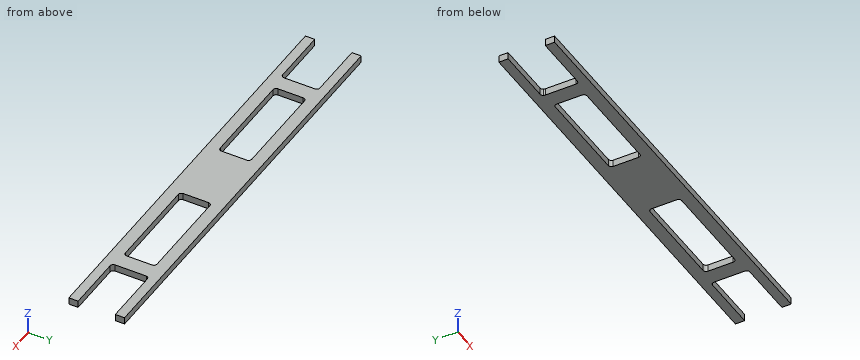
Autodesk Inventor part; units mm, degrees
ref_plane "YZ Plane" through (0, 0, 0) normal (1, 0, 0) x (0, 1, 0)
ref_plane "XZ Plane" through (0, 0, 0) normal (0, 1, 0) x (-1, 0, 0)
ref_plane "XY Plane" through (0, 0, 0) normal (0, 0, 1) x (1, 0, 0)
sketch "Sketch1" plane through (0, 0, 0) normal (0, 0, 1) x (1, 0, 0)
  line L0 (282.4312, 43.9885) -> (-286.5277, 43.9885)
  line L1 (-286.5288, -32.1915) -> (282.4312, -32.1915)
  line L2 (-286.5277, 43.9885) -> (-286.5277, 31.2885)
  line L3 (-286.5288, -19.4915) -> (-286.5288, -32.1915)
  line L4 (282.4312, 31.3086) -> (282.4312, 43.9885)
  line L5 (282.4312, -19.4915) -> (282.4312, -32.1915)
  arc A0 (-205.7269, 29.0424) -> (-209.4741, 31.2885) centre (-209.4741, 27.0395) ccw
  arc A1 (-205.2441, 26.6389) -> (-205.7269, 29.0424) centre (-209.4741, 27.0395) ccw
  arc A2 (-209.4751, -19.4915) -> (-205.2441, -15.2625) centre (-209.4741, -15.2615) ccw
  arc A3 (-179.9924, 27.4418) -> (-183.6588, 23.2495) centre (-179.4288, 23.2495) ccw
  arc A4 (-183.6588, -11.4325) -> (-179.4288, -15.6625) centre (-179.4288, -11.4325) ccw
  arc A5 (-48.2006, 23.2495) -> (-52.4306, 27.4418) centre (-52.4304, 23.2118) ccw
  arc A6 (-52.9924, -15.6625) -> (-48.2006, -11.4325) centre (-52.4304, -11.47) ccw
  line L6 (-52.4306, 27.4418) -> (-179.9924, 27.4418)
  line L7 (-52.9924, -15.6625) -> (-179.4288, -15.6625)
  line L8 (-48.2006, -11.4325) -> (-48.2006, 23.2495)
  line L9 (-183.6588, -11.4325) -> (-183.6588, 23.2495)
  arc A7 (205.3642, 31.3086) -> (201.1322, 27.4399) centre (205.3642, 27.0596) ccw
  arc A8 (201.1322, -15.2425) -> (205.3812, -19.4915) centre (205.3812, -15.2425) ccw
  line L10 (201.1322, -15.2425) -> (201.1322, 23.2474)
  line L11 (201.1322, 23.2474) -> (201.1322, 27.4399)
  line L12 (282.4312, 31.3086) -> (205.3642, 31.3086)
  line L13 (282.4312, -19.4915) -> (205.3812, -19.4915)
  line L14 (-286.5288, -19.4915) -> (-209.4751, -19.4915)
  line L15 (-286.5277, 31.2885) -> (-209.4741, 31.2885)
  line L16 (-205.2441, 26.6389) -> (-205.2441, -15.2625)
  arc A9 (48.2152, 27.4415) -> (43.9852, 23.2115) centre (48.2152, 23.2115) ccw
  arc A10 (43.9852, -11.4145) -> (48.2152, -15.6445) centre (48.2152, -11.4145) ccw
  arc A11 (179.5472, 23.2115) -> (175.3172, 27.4415) centre (175.3172, 23.2115) ccw
  arc A12 (175.3172, -15.6445) -> (179.5472, -11.4145) centre (175.3172, -11.4145) ccw
  line L17 (48.2152, 27.4415) -> (175.3172, 27.4415)
  line L18 (48.2152, -15.6445) -> (175.3172, -15.6445)
  line L19 (43.9852, 23.2115) -> (43.9852, -11.4145)
  line L20 (179.5472, 23.2115) -> (179.5472, -11.4145)
  point P0 (0, 0)
  point P1 (0, 0)
  dimension "d0" = 135.4582
  dimension "d1" = 43.1043
  dimension "d2" = 16.5467
  dimension "d3" = 16.529
  dimension "d4" = 21.5853
  dimension "d5" = 92.1858
extrude "Extrusion1" add sketch "Sketch1" along normal blind 9.525
properties part number "top"
Design review of the part built by this model. Coordinates are the model's own, in mm. Coordinates: 2 decimals unless noted, no trailing zeros. Loops run counter-clockwise (first coordinate to the right, second up) from the corner with the lowest first, then second, coordinate; pieces in that order, holes last. Notation, with made-up numbers: M 74.25,36.25 L 83.25,36.25 A30 cw 83.25,67.25 Z; hole C 51.25,42.5 d11. An arc over 180 degrees is marked long. Answer as CSV lines item,"result".
Item 1: For P1, Ø3, axis at y = 1, z = 3.5, coming from the -X side; P2, Ø5, axis at y = 13.5, z = 7.5, coming from the +X side, all flat-tipped, find the tip position at first contact; note any pin that passes through.
Answer list:
P1,"x = -205.24"
P2,"x = 201.13"
Item 2: Add section A-A on y = 8. State the section outline as (x, z) points (3 decimals), plus the area to 3 significant figures.
Answer list:
outline,"M -205.244,0 L -183.659,0 L -183.659,9.525 L -205.244,9.525 Z; M -48.201,0 L 43.985,0 L 43.985,9.525 L -48.201,9.525 Z; M 179.547,0 L 201.132,0 L 201.132,9.525 L 179.547,9.525 Z"
area,"1,290 mm²"
Item 3: Add section B-B on x = -242. State the section outline as (y, z) points (1 decimal), plus the area to 3 significant figures.
Answer list:
outline,"M -32.2,0 L -19.5,0 L -19.5,9.5 L -32.2,9.5 Z; M 31.3,0 L 44,0 L 44,9.5 L 31.3,9.5 Z"
area,"242 mm²"
Item 4: For probe 1 along X at (y, z) = (14, 7.5); probe 2 along Y at (x, z) = (-109.5, 4.5); probe 3 along X at (y, z) = (-12, 7.5), list the stretches that pass through material, from the lowest coordinate up.
Answer list:
probe 1,"-205.24 to -183.66, -48.2 to 43.99, 179.55 to 201.13"
probe 2,"-32.19 to -15.66, 27.44 to 43.99"
probe 3,"-205.24 to -183.62, -48.23 to 44.03, 179.51 to 201.13"
Item 5: Add section D-D on x = 141. State the section outline as (y, z) points (1 decimal), plus the area to 3 significant figures.
Answer list:
outline,"M -32.2,0 L -15.6,0 L -15.6,9.5 L -32.2,9.5 Z; M 27.4,0 L 44,0 L 44,9.5 L 27.4,9.5 Z"
area,"315 mm²"
Item 6: Add section C-C on z = 1.5. Count the separate pieces of the cut face and the enclosed holes in it, plus the area to 3 significant figures.
Answer list:
separate pieces,"1"
enclosed holes,"2"
area,"23,500 mm²"
